from build123d import *

# Parameters (mm, degrees)
SKETCH1_W           = 58.42
SKETCH1_H           = 50.038
BOSS_EXTRUDE1_DEPTH = 6.35
SKETCH2_R           = 1.143
CUT_EXTRUDE1_DEPTH  = 3.81
SKETCH3_R           = 1.143
CUT_EXTRUDE2_DEPTH  = 3.81


with BuildPart() as part:
    # Sketch1 → Boss-Extrude1 (new body)
    with BuildSketch(Plane.XY):
        with Locations((0, 25.019)):
            Rectangle(SKETCH1_W, SKETCH1_H)
        Polygon((-25.4, 46.228), (-25.4, 3.81), (-5.715, 3.81), align=None, mode=Mode.SUBTRACT)
        Polygon((1.905, 46.228), (1.905, 3.81), (21.59, 46.228), align=None, mode=Mode.SUBTRACT)
        Polygon((-21.59, 46.228), (-1.905, 3.81), (-1.905, 46.228), align=None, mode=Mode.SUBTRACT)
        Polygon((5.715, 3.81), (25.4, 46.228), (25.4, 3.81), align=None, mode=Mode.SUBTRACT)
    extrude(amount=BOSS_EXTRUDE1_DEPTH)

    # Sketch2 → Cut-Extrude1 (cut)
    with BuildSketch(Plane(origin=(0, 0, 0), x_dir=(1, 0, 0), z_dir=(0, 1, 0))):
        with Locations((-18.0975, -3.175)):
            Circle(SKETCH2_R)
        with Locations((-13.0175, -3.175)):
            Circle(SKETCH2_R)
        with Locations((18.0975, -3.175)):
            Circle(SKETCH2_R)
        with Locations((13.0175, -3.175)):
            Circle(SKETCH2_R)
    extrude(amount=CUT_EXTRUDE1_DEPTH, mode=Mode.SUBTRACT)

    # Sketch3 → Cut-Extrude2 (cut)
    with BuildSketch(Plane(origin=(0, 50.038, 0), x_dir=(1, 0, 0), z_dir=(0, 1, 0))):
        with Locations((-14.2875, -3.175)):
            Circle(SKETCH3_R)
        with Locations((-9.2075, -3.175)):
            Circle(SKETCH3_R)
        with Locations((9.2075, -3.175)):
            Circle(SKETCH3_R)
        with Locations((14.2875, -3.175)):
            Circle(SKETCH3_R)
    extrude(amount=-CUT_EXTRUDE2_DEPTH, mode=Mode.SUBTRACT)


solid = part.part
Verification items for the finished model (mm, model axes). A direction names the side the tool comes from. Give positions to 0.01 mm unless a question says otherwise; leave off trailing zeros. Write each loop counter-clockwise with the first axis right and the second up, starting at its lowest first coordinate (ties: lowest second). Pieces come first, ordered by that corner, then holes.
(1) Cross-section at A-A (x = -4). Enter the section's corners in (y, z), plus the area to 3 significant figures.
(2) Cross-section at D-D (x = 24). Enter the section's corners in (y, z), plus the area to 3 significant figures.
(3) Gauge pin test, flat ends, axial feed: pin 1 (3.5 mm diameter, centred on x = 9.21, z = 3.18, fed in from +Y); pin 2 (6 mm diameter, centred on x = -18.5, y = 7, fed in from +Z). Record the tip position at first contact, or that the pin passes through.
(4) Material ranges on line 1 (X direction, y = 37, z = 5.5) (3 decimals); line 2 (Y direction, x = 21.5, z = 1.25); line 3 (X direction, y = 17, z = 6.25) (3 decimals), recorded low to high.
(5) Cross-section at C-C (x = -18). Enter the section's corners in (y, z), plus the area to 3 significant figures.
(6) Access from +Z, -Z, +X, -X, +Y, -Y to the whole of each face (thin tool, end or side, straight path). Record for faces 1 (the face through (-19.24, 1.88, 3.12)), 2 (the face through (13.146, 48.16, 3.125)), 3 (the face through (-12, 46.228, 3)).
(7) Mould release check, pull along X, two halves, no side actions. Record for faces 4 (the face through (-15.42, 24.72, 3.13)), 5 (the face through (0, 25, 0)), 6 (the face through (-29.21, 25, 3)), 7 (the face through (29.21, 25, 3)): +X half, -X half, draft (parallel to the pull), parting line (faces both ways), or undercut.
(8) Cross-section at B-B (y = 42.5). Enter the section's corners in (x, z) (3 decimals), plus the area to 3 significant figures.
Worked out:
1. outline: (0, 0) - (8.32, 0) - (8.32, 6.35) - (0, 6.35) - close; (46.23, 0) - (50.04, 0) - (50.04, 6.35) - (46.23, 6.35) - close
1. area: 77.1 mm2
2. outline: (0, 0) - (3.81, 0) - (3.81, 6.35) - (0, 6.35) - close; (43.21, 0) - (50.04, 0) - (50.04, 6.35) - (43.21, 6.35) - close
2. area: 67.5 mm2
3. pin 1: stops at y = 50.04
3. pin 2: passes through
4. line 1: x = -29.21 to -25.4, -21.118 to -17.308, -1.905 to 1.905, 17.308 to 21.118, 25.4 to 29.21
4. line 2: y = 0 to 3.81, 37.82 to 46.03, 46.23 to 50.04
4. line 3: x = -29.21 to -25.4, -11.836 to -8.026, -1.905 to 1.905, 8.026 to 11.836, 25.4 to 29.21
5. outline: (0, 0) - (3.81, 0) - (3.81, 2.04) - (0, 2.04) - close; (0, 4.31) - (3.81, 4.31) - (3.81, 6.35) - (0, 6.35) - close; (30.28, 0) - (38.49, 0) - (38.49, 6.35) - (30.28, 6.35) - close; (46.23, 0) - (50.04, 0) - (50.04, 6.35) - (46.23, 6.35) - close
5. area: 91.8 mm2
6. face 1: -Y
6. face 2: +Y
6. face 3: +Z, -Z
7. face 4: undercut
7. face 5: draft
7. face 6: -X half
7. face 7: +X half
8. outline: (-29.21, 0) - (-25.4, 0) - (-25.4, 6.35) - (-29.21, 6.35) - close; (-23.67, 0) - (-19.86, 0) - (-19.86, 6.35) - (-23.67, 6.35) - close; (-1.905, 0) - (1.905, 0) - (1.905, 6.35) - (-1.905, 6.35) - close; (19.86, 0) - (23.67, 0) - (23.67, 6.35) - (19.86, 6.35) - close; (25.4, 0) - (29.21, 0) - (29.21, 6.35) - (25.4, 6.35) - close
8. area: 121 mm2
